Read the model definition and answer for the solid it produces. Units are mm, in the model's axes. A direction names the side the tool comes from. Give positions to 0.01 mm unless a question says otherwise; leave off trailing zeros. Loops run counter-clockwise (first coordinate to the right, second up) from the corner with the lowest first, then second, coordinate; pieces in that order, holes last. Notation, with made-up numbers: (62.25, 68.25) - (74.25, 68.25) arc R5 cw to (74.25, 72.25) - close; hole circle Ø6 at (73.25, -1.75). An arc over 180 degrees is marked (long way). Write each question's results on one line, items separated by ' | '. Start each with the question number.
Q1. For faces 5 (the cylindrical face through (0.5, 0.1, -2.4)), 6 (the cylindrical face through (6.45, 0.35, -9.06)), determine the directions among +Z, -Z, +X, -X, +Y, -Y from which every point of the face is accessible in a straight line to the end or side of a thin tool.
Q2. Given pin 1 (5 mm diameter, centred on x = -2, z = 7.5, fed in from +Y); pin 2 (1.9 mm diameter, centred on y = 0, z = 2.5, fed in from +X), each flat-ended and moving along its own axis, determine where each tip first touches the part or whether it passes through.
Q3. The part is cut by section A-A, the plane x = -2. Write down the section's boundary in (y, z), plus the area to 3 significant figures.
Q4. Determine the mould class of faces 1 (the flat face through (0, -4, 0)), 2 (the conical face through (2.206, -0.06, 2.229)), 3 (the conical face through (2.21, 0.13, -7.75)), 4 (the flat face through (0, 4, 0)) for opening direction Y: +Y half, -Y half, draft (parallel to the pull), parting line (faces both ways), or undercut.
Q5. Find the intervals of material crossed by line 1 (Z direction, x = 6, y = 0); line 2 (Z direction, x = -2, y = 2); line 3 (Y direction, x = 5.25, z = -7.5), in increasing order. Write a range as from..to.
Q6. The part is cut by section B-B, the plane z = -4.5. Write down the section's boundary in (x, y).
Q7. The part is cut by section C-C, the plane y = 2.5. Write down the section's boundary in (x, z), plus the area to 3 significant figures.
Q8. The part is cut by section D-D, the plane x = 7.5. Write down the section's boundary in (y, z).
```python
from build123d import *

# Parameters (mm, degrees)
F0_W     = 20
F0_H     = 25
F1_DEPTH = 4
F3_D     = 4
F4_D     = 5
F6_D     = 3.2
F6_DEPTH = 7
F6_TIP   = 0.9613769904


with BuildPart() as f1:
    # F0 (on Front) → F1 (new body, symmetric)
    with BuildSketch(Plane.XZ):
        Rectangle(F0_W, F0_H)
    extrude(amount=F1_DEPTH, both=True)

    # F3 (through all)
    with Locations(Plane.XZ.offset(4)):
        with Locations((-2, 7.5)):
            Hole(F3_D / 2)

    # F4 (through all)
    with Locations(Plane.XZ.offset(4)):
        with Locations((-2, -2.5)):
            Hole(F4_D / 2)

    # F6
    with Locations(Plane.YZ.offset(10)):
        with Locations((0, 2.5), (0, -7.5)):
            Hole(F6_D / 2, depth=F6_DEPTH)
            with Locations((0, 0, -(F6_DEPTH + F6_TIP / 2))):  # 118° drill point
                Cone(0, F6_D / 2, F6_TIP, mode=Mode.SUBTRACT)


solid = f1.part
```
Check sheet entries:
1) face 5: +Y, -Y | face 6: +X
2) pin 1: stops at y = 4 | pin 2: stops at x = 2.61
3) outline: (-4, -12.5) - (4, -12.5) - (4, -5) - (-4, -5) - close; (-4, 0) - (4, 0) - (4, 5.5) - (-4, 5.5) - close; (-4, 9.5) - (4, 9.5) - (4, 12.5) - (-4, 12.5) - close | area: 128 mm^2
4) face 1: -Y half | face 2: undercut | face 3: undercut | face 4: +Y half
5) line 1: z = -12.5..-9.1, -5.9..0.9, 4.1..12.5 | line 2: z = -12.5..-5, 0..5.5, 9.5..12.5 | line 3: y = -4..-1.6, 1.6..4
6) outline: (-10, -4) - (-3.5, -4) - (-3.5, 4) - (-10, 4) - close; (-0.5, -4) - (10, -4) - (10, 4) - (-0.5, 4) - close
7) outline: (-10, -12.5) - (10, -12.5) - (10, 12.5) - (-10, 12.5) - close; hole circle Ø5 at (-2, -2.5); hole circle Ø4 at (-2, 7.5) | area: 468 mm^2
8) outline: (-4, -12.5) - (4, -12.5) - (4, 12.5) - (-4, 12.5) - close; hole circle Ø3.2 at (0, -7.5); hole circle Ø3.2 at (0, 2.5)
